from build123d import *

# Parameters (mm, degrees)
BOSS_EXTRUDE1_DEPTH = 65
BOSS_EXTRUDE2_DEPTH = 129.75
SKETCH5_W           = 1.39
SKETCH5_H           = 3.378
CUT_EXTRUDE1_DEPTH  = 0.25
SKETCH8_R           = 0.5
CUT_EXTRUDE2_DEPTH  = 2
BOSS_EXTRUDE3_DEPTH = 0.0625
SKETCH11_W          = 12.625
SKETCH11_H          = 5.25
CUT_EXTRUDE4_DEPTH  = 11.75
SKETCH12_W          = 12.625
SKETCH12_H          = 5.25
SKETCH12_W_2        = 12.025
SKETCH12_H_2        = 4.65
BOSS_EXTRUDE4_DEPTH = 8.875
SKETCH13_W          = 11.525
SKETCH13_H          = 1.56
BOSS_EXTRUDE5_DEPTH = 8.875
CUT_EXTRUDE5_DEPTH  = 10
SKETCH17_W          = 5.5
SKETCH17_H          = 0.125
BOSS_EXTRUDE6_DEPTH = 8.1
BOSS_EXTRUDE7_START = 8
BOSS_EXTRUDE7_DEPTH = 8


with BuildPart() as part:
    # Sketch1 → Boss-Extrude1 (new, symmetric)
    with BuildSketch(Plane(origin=(0, 0, 0), x_dir=(1, 0, 0), z_dir=(0, 1, 0))):
        with BuildLine():
            Line((-28.45, 7.05), (28.45, 7.05))
            ThreePointArc((28.45, 7.05), (35.5, 0), (28.45, -7.05))
            Line((28.45, -7.05), (-28.45, -7.05))
            ThreePointArc((-28.45, -7.05), (-35.5, 0), (-28.45, 7.05))
        make_face()
        with BuildLine():
            Line((-28.45, 6.38), (28.45, 6.38))
            ThreePointArc((28.45, 6.38), (34.83, 0), (28.45, -6.38))
            Line((28.45, -6.38), (-28.45, -6.38))
            ThreePointArc((-28.45, -6.38), (-34.83, 0), (-28.45, 6.38))
        make_face(mode=Mode.SUBTRACT)
    extrude(amount=BOSS_EXTRUDE1_DEPTH, both=True)

    # Sketch2 → Boss-Extrude2 (add)
    with BuildSketch(Plane(origin=(0, 64.875, 0), x_dir=(1, 0, 0), z_dir=(0, 1, 0))):
        with BuildLine():
            Line((-28.45, -6.38), (28.45, -6.38))
            ThreePointArc((28.45, -6.38), (34.83, 0), (28.45, 6.38))
            Line((28.45, 6.38), (-28.45, 6.38))
            ThreePointArc((-28.45, 6.38), (-34.83, 0), (-28.45, -6.38))
        make_face()
    extrude(amount=-BOSS_EXTRUDE2_DEPTH)

    # Sketch5 → Cut-Extrude1 (cut)
    with BuildSketch(Plane(origin=(0, 0, -7.05), x_dir=(-1, 0, 0), z_dir=(0, 0, -1))):
        Polygon((3.047959184, -38.5), (4.369798182, -38.5), (4.369798182, -33), (3.039285714, -33), align=None)
        with BuildLine():
            Line((-4.125, -33), (-4.125, -38.5))
            Line((-4.125, -38.5), (-2.775, -38.5))
            Line((-2.775, -38.5), (-2.775, -34.15))
            Line((-2.775, -34.15), (-0.025, -34.15))
            ThreePointArc((-0.025, -34.15), (0.481245093, -34.446327571), (0.675, -35))
            Line((0.675, -35), (0.675, -38.5))
            Line((0.675, -38.5), (1.975, -38.5))
            Line((1.975, -38.5), (1.975, -34.330645161))
            add(Edge.make_bspline(
                [(1.975, -34.330645161), (1.946635107, -34.301634388), (1.95702187, -34.248224197), (1.948979592, -34.215322581), (1.924253679, -34.114166856), (1.916519719, -34.042472973), (1.870918367, -33.949193548), (1.843725239, -33.893568896), (1.820050271, -33.836269814), (1.792857143, -33.780645161), (1.758600377, -33.710571549), (1.699108422, -33.633824398), (1.645408163, -33.576612903), (1.280199443, -33.187524707), (1.016815103, -33.047701351), (0.457142857, -33)],
                knots=[0, 0, 0, 0, 1, 1, 1, 2, 2, 2, 3, 3, 3, 4, 4, 4, 5, 5, 5, 5], degree=3))
            Line((0.457142857, -33), (-4.125, -33))
        make_face()
        with Locations((-1.06, -36.811)):
            Rectangle(SKETCH5_W, SKETCH5_H)
    extrude(amount=-CUT_EXTRUDE1_DEPTH, mode=Mode.SUBTRACT)

    # Sketch8 → Cut-Extrude2 (cut)
    with BuildSketch(Plane(origin=(0, 64.875, 0), x_dir=(1, 0, 0), z_dir=(0, 1, 0))):
        with Locations(Location((-14, 0, 0), (0, 0, 270))):
            Circle(SKETCH8_R)
        with Locations(Location((-10.25, 0, 0), (0, 0, 270))):
            Circle(SKETCH8_R)
        with Locations(Location((-6.5, 0, 0), (0, 0, 270))):
            Circle(SKETCH8_R)
        with Locations(Location((-2.75, 0, 0), (0, 0, 270))):
            Circle(SKETCH8_R)
    extrude(amount=-CUT_EXTRUDE2_DEPTH, mode=Mode.SUBTRACT)

    # Sketch9 → Boss-Extrude3 (add)
    with BuildSketch(Plane(origin=(0, 64.875, 0), x_dir=(1, 0, 0), z_dir=(0, 1, 0))):
        with BuildLine():
            Line((-28.375, 1.4375), (-20.25, 1.4375))
            ThreePointArc((-20.25, 1.4375), (-18.8125, 0), (-20.25, -1.4375))
            Line((-20.25, -1.4375), (-28.375, -1.4375))
            ThreePointArc((-28.375, -1.4375), (-29.8125, 0), (-28.375, 1.4375))
        make_face()
    extrude(amount=BOSS_EXTRUDE3_DEPTH)

    # Sketch11 → Cut-Extrude4 (cut)
    with BuildSketch(Plane(origin=(0, 64.875, 0), x_dir=(1, 0, 0), z_dir=(0, 1, 0))):
        with Locations((21.0625, 0)):
            Rectangle(SKETCH11_W, SKETCH11_H)
    extrude(amount=-CUT_EXTRUDE4_DEPTH, mode=Mode.SUBTRACT)

    # Sketch12 → Boss-Extrude4 (add)
    with BuildSketch(Plane(origin=(0, 53.125, 0), x_dir=(1, 0, 0), z_dir=(0, 1, 0))):
        with Locations((21.0625, 0)):
            Rectangle(SKETCH12_W, SKETCH12_H)
        with Locations((21.0625, 0)):
            Rectangle(SKETCH12_W_2, SKETCH12_H_2, mode=Mode.SUBTRACT)
    extrude(amount=BOSS_EXTRUDE4_DEPTH)

    # Sketch13 → Boss-Extrude5 (add)
    with BuildSketch(Plane(origin=(0, 53.125, 0), x_dir=(1, 0, 0), z_dir=(0, 1, 0))):
        with Locations((21.0625, -1.17)):
            Rectangle(SKETCH13_W, SKETCH13_H)
    extrude(amount=BOSS_EXTRUDE5_DEPTH)

    # Sketch16 → Cut-Extrude5 (cut)
    with BuildSketch(Plane(origin=(0, 64.875, 0), x_dir=(1, 0, 0), z_dir=(0, 1, 0))):
        with BuildLine():
            Line((4.111130468, 1.08), (9.338869532, 1.08))
            ThreePointArc((9.338869532, 1.08), (9.462834417, 1.053189874), (9.56464254, 0.977551382))
            Line((9.56464254, 0.977551382), (10.275773008, 0.164830848))
            ThreePointArc((10.275773008, 0.164830848), (10.330830823, 0.072797467), (10.35, -0.032720535))
            Line((10.35, -0.032720535), (10.35, -1.08))
            Line((10.35, -1.08), (3.1, -1.08))
            Line((3.1, -1.08), (3.1, -0.032720535))
            ThreePointArc((3.1, -0.032720535), (3.119169177, 0.072797467), (3.174226992, 0.164830848))
            Line((3.174226992, 0.164830848), (3.88535746, 0.977551382))
            ThreePointArc((3.88535746, 0.977551382), (3.987165583, 1.053189874), (4.111130468, 1.08))
        make_face()
    extrude(amount=-CUT_EXTRUDE5_DEPTH, mode=Mode.SUBTRACT)

    # Sketch17 → Boss-Extrude6 (add)
    with BuildSketch(Plane(origin=(0, 54.875, 0), x_dir=(1, 0, 0), z_dir=(0, 1, 0))):
        with Locations((6.725, -0.7675)):
            Rectangle(SKETCH17_W, SKETCH17_H)
    extrude(amount=BOSS_EXTRUDE6_DEPTH)

    # Sketch18 → Boss-Extrude7 (add)
    with BuildSketch(Plane(origin=(0, 54.875, 0), x_dir=(1, 0, 0), z_dir=(0, 1, 0)).offset(BOSS_EXTRUDE7_START)):
        with BuildLine():
            Line((3.1, -1.08), (10.35, -1.08))
            Line((10.35, -1.08), (10.35, -0.032720535))
            ThreePointArc((10.35, -0.032720535), (10.330830823, 0.072797467), (10.275773008, 0.164830848))
            Line((10.275773008, 0.164830848), (9.56464254, 0.977551382))
            ThreePointArc((9.56464254, 0.977551382), (9.462834417, 1.053189874), (9.338869532, 1.08))
            Line((9.338869532, 1.08), (4.111130468, 1.08))
            ThreePointArc((4.111130468, 1.08), (3.987165583, 1.053189874), (3.88535746, 0.977551382))
            Line((3.88535746, 0.977551382), (3.174226992, 0.164830848))
            ThreePointArc((3.174226992, 0.164830848), (3.119169177, 0.072797467), (3.1, -0.032720535))
            Line((3.1, -0.032720535), (3.1, -1.08))
        make_face()
        with BuildLine():
            Line((3.225, -0.032720535), (3.225, -0.955))
            Line((3.225, -0.955), (10.225, -0.955))
            Line((10.225, -0.955), (10.225, -0.032720535))
            ThreePointArc((10.225, -0.032720535), (10.21381798, 0.028831633), (10.181700922, 0.082517772))
            Line((10.181700922, 0.082517772), (9.470570454, 0.895238306))
            ThreePointArc((9.470570454, 0.895238306), (9.411182381, 0.93936076), (9.338869532, 0.955))
            Line((9.338869532, 0.955), (4.111130468, 0.955))
            ThreePointArc((4.111130468, 0.955), (4.038817619, 0.93936076), (3.979429546, 0.895238306))
            Line((3.979429546, 0.895238306), (3.268299078, 0.082517772))
            ThreePointArc((3.268299078, 0.082517772), (3.23618202, 0.028831633), (3.225, -0.032720535))
        make_face(mode=Mode.SUBTRACT)
    extrude(amount=-BOSS_EXTRUDE7_DEPTH)


solid = part.part
Design review of the part built by this model. Coordinates are the model's own, in mm. A direction names the side the tool comes from. Coordinates: 2 decimals unless noted, no trailing zeros. Loops run counter-clockwise (first coordinate to the right, second up) from the corner with the lowest first, then second, coordinate; pieces in that order, holes last.
Item 1: Add section B-B (y = 19). Write out the cut boundary in (x, z).
Completed:
outline: (-28.45, -7.05) - (28.45, -7.05) arc R7.05 ccw to (28.45, 7.05) - (-28.45, 7.05) arc R7.05 ccw to start
Item 2: For faces 1 (the flat face through (0, -64.875, 0)), 2 (the flat face through (0.2, 65, 6.8)), 3 (the flat face through (15.05, 58, 0)), list the 3-axis set-ups (+Z, -Z, +X, -X, +Y, -Y) from which the entire face can be reached by the end or side of a thin tool; tool diameter is ignored.
Completed:
face 1: -Y
face 2: +Z, -Z, +X, -X, +Y
face 3: +Y
Item 3: Clearance check with flat-ended pins moving along their axes: pin 1 (4 mm diameter, centred on x = 22, z = 1, fed in from +Y) (3 decimals); pin 2 (1 mm diameter, centred on x = -3, z = -5.5, fed in from -Y) (3 decimals); pin 3 (1.5 mm diameter, centred on y = -14, z = 2.5, fed in from +X). State where each tip first meets the part, or that it passes through.
Completed:
pin 1: stops at y = 64.875
pin 2: stops at y = -64.875
pin 3: stops at x = 35.28
Item 4: Add section A-A (x = 20). Write out the cut boundary in (y, z) (3 decimals), and give its area (3 significant figures).
Completed:
outline: (-65, -7.05) - (65, -7.05) - (65, -6.38) - (64.875, -6.38) - (64.875, -2.625) - (62, -2.625) - (62, -2.325) - (53.125, -2.325) - (53.125, 0.39) - (62, 0.39) - (62, 1.95) - (53.125, 1.95) - (53.125, 2.325) - (62, 2.325) - (62, 2.625) - (64.875, 2.625) - (64.875, 6.38) - (65, 6.38) - (65, 7.05) - (-65, 7.05) - (-65, 6.38) - (-64.875, 6.38) - (-64.875, -6.38) - (-65, -6.38) - close
area: 1,790 mm2
Item 5: Draft analysis for pull direction Z (two halves, no side actions). For faces 4 (the cylindrical face through (-35.5, 0.91, 0.16)), 5 (the flat face through (0.2, -65, 6.8)), 6 (the flat face through (0, 1, 7.05)), 7 (the flat face through (21, 58, -2.325)), state which applies: pulls with the +Z half, pulls with the -Z half, needs draft (parallel to the pull), parting line crosses it, or undercut.
Completed:
face 4: parting line crosses it
face 5: needs draft
face 6: pulls with the +Z half
face 7: undercut
Item 6: Wall thickness on L1, parallel to Y at x = 0, z = -0.25 (3 decimals); L2, parallel to Z at x = -10, y = 63; L3, parallel to X at y = -20.5, z = 3: over which ranges is each line inside the solid? List them lowest first.
Completed:
L1: y = -64.875 to 64.875
L2: z = -7.05 to -0.43, 0.43 to 7.05
L3: x = -34.83 to 34.83
